```python
from build123d import *

# Parameters (mm, degrees)
SKETCH1_R           = 7.5
BOSS_EXTRUDE1_DEPTH = 15


with BuildPart() as part:
    # Sketch1 → Boss-Extrude1 (new, symmetric)
    with BuildSketch(Plane.XY):
        Polygon((-185, -225), (-185, -15), (185, -15), (185, -225), (215, -225), (215, -15), (215, 15), (-215, 15), (-215, -15), (-215, -225), align=None)
        with Locations((-200, -210)):
            Circle(SKETCH1_R, mode=Mode.SUBTRACT)
        with Locations((200, -210)):
            Circle(SKETCH1_R, mode=Mode.SUBTRACT)
    extrude(amount=BOSS_EXTRUDE1_DEPTH, both=True)


solid = part.part
```
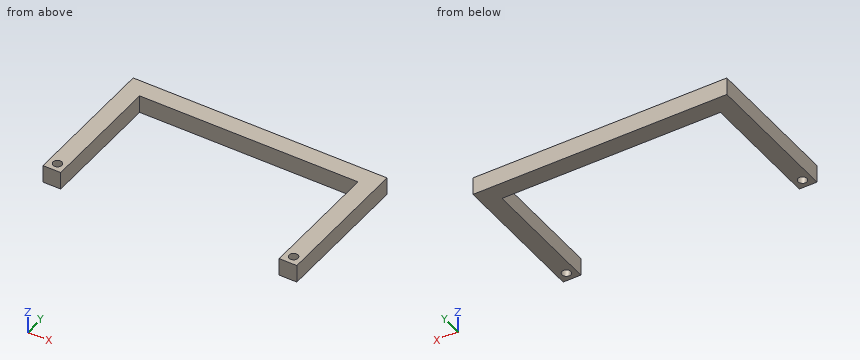
Check sheet for the modelled part. Datum: model origin and axes. Units: mm. Coordinates: 2 decimals unless noted, no trailing zeros. Write each loop counter-clockwise with the first axis right and the second up, starting at its lowest first coordinate (ties: lowest second). Pieces come first, ordered by that corner, then holes. Notation, with made-up numbers: (-36, 85) -> (-14, 85) arc R22 ccw to (-14, 113) -> close; hole circle Ø8 at (-31, -16.5). An arc over 180 degrees is marked (long way). Use a Markdown table: item, result.
1. Sectioned sample at B-B (y = -59.5). Enter the section's corners in (x, z), plus the area to 3 significant figures.
Reported:
| item | result |
|---|---|
| outline | (-215, -15) -> (-185, -15) -> (-185, 15) -> (-215, 15) -> close; (185, -15) -> (215, -15) -> (215, 15) -> (185, 15) -> close |
| area | 1,800 mm2 |
2. Sectioned sample at D-D (y = -210). Enter the section's corners in (x, z).
Reported:
| item | result |
|---|---|
| outline | (-215, -15) -> (-207.5, -15) -> (-207.5, 15) -> (-215, 15) -> close; (-192.5, -15) -> (-185, -15) -> (-185, 15) -> (-192.5, 15) -> close; (185, -15) -> (192.5, -15) -> (192.5, 15) -> (185, 15) -> close; (207.5, -15) -> (215, -15) -> (215, 15) -> (207.5, 15) -> close |
3. Scan lines: line 1 along Y through (x, z) = (200, -4); line 2 along X through (y, z) = (-89.5, 5); line 3 along Y through (x, z) = (-11.5, -11.5). Record each from-to range of solid material in increasing order.
Reported:
| item | result |
|---|---|
| line 1 | y = -225 to -217.5, -202.5 to 15 |
| line 2 | x = -215 to -185, 185 to 215 |
| line 3 | y = -15 to 15 |
4. Go/stop test with a flat-tipped pin: pin 1 Ø1.5 at (x, z) = (78, 3.5) entering from -Y. Record where the tip stops, or that it passes through.
Reported:
| item | result |
|---|---|
| pin 1 | stops at y = -15 |
5. Sectioned sample at A-A (x = 200). Enter the section's corners in (y, z), plus the area to 3 significant figures.
Reported:
| item | result |
|---|---|
| outline | (-225, -15) -> (-217.5, -15) -> (-217.5, 15) -> (-225, 15) -> close; (-202.5, -15) -> (15, -15) -> (15, 15) -> (-202.5, 15) -> close |
| area | 6,750 mm2 |
6. Sectioned sample at C-C (z = 5.25). Enter the section's corners in (x, y).
Reported:
| item | result |
|---|---|
| outline | (-215, -225) -> (-185, -225) -> (-185, -15) -> (185, -15) -> (185, -225) -> (215, -225) -> (215, 15) -> (-215, 15) -> close; hole circle Ø15 at (-200, -210); hole circle Ø15 at (200, -210) |
